The listing builds one solid part. Answer for the finished solid, in the listing's coordinates (mm). A direction names the side the tool comes from. Round coordinates to 2 decimals unless told otherwise and drop trailing zeros. Write each loop counter-clockwise with the first axis right and the second up, starting at its lowest first coordinate (ties: lowest second). Pieces come first, ordered by that corner, then holes. Notation, with made-up numbers: (89.25, 46.25) - (116.25, 46.25) arc R24 cw to (116.25, 74.25) - close; hole circle Ø2 at (68, -16.5). An arc over 180 degrees is marked (long way). Answer as CSV lines item,"result". Start each with the question number.
Item 1: For a pull along Y with two mould halves and no side action, classify faces 1 (the flat face through (-26, 76.809, 1)), 2 (the cylindrical face through (-18.75, 30.73, 4.5)), 3 (the cylindrical face through (-23.75, 24.89, 4.5)) as pulls with the +Y half, pulls with the -Y half, needs draft (parallel to the pull), parting line crosses it, or undercut.
Item 2: Flat-ended cylindrical pins translate along their axes: pin 1 (2 mm diameter, centred on x = -15.5, z = 1, fed in from +Y); pin 2 (4 mm diameter, centred on x = -21.25, y = 26.81, fed in from +Z); pin 3 (4 mm diameter, centred on x = -16, y = 59, fed in from -Z); pin 4 (1.5 mm diameter, centred on x = -14.5, z = 1.5, fed in from +Y). Find the tip coordinate at first contact, or state that the pin passes through.
Item 3: A cutting plane is placed at A-A on y = 60. Determine the outline of the cut face in (x, z), and give its area (3 significant figures).
Item 4: Straight lines are drawn through the part: line 1 along Y through (x, z) = (-21.25, 2.3); line 2 along Y through (x, z) = (-21.25, 4.75); line 3 along Y through (x, z) = (-20, 1.25). For each, find the intervals that lie inside material, in ascending order. Write a range as [from, to].
Item 5: A cutting plane is placed at B-B on x = -14. Determine the outline of the cut face in (y, z).
Item 6: Which of the six approach directions +Z, -Z, +X, -X, +Y, -Y give full straight-line access (tool end or side, diameter ignored) to faces 4 (the cylindrical face through (-21.47, 16.81, 1.48)), 5 (the flat face through (-23, 26, 3))?
```python
from build123d import *

# Parameters (mm, degrees)
BOSS_EXTRUDE1_DEPTH = 3
SKETCH2_R           = 4.65
SKETCH2_R_2         = 3.15
BOSS_EXTRUDE2_DEPTH = 3.044394089
SKETCH3_R           = 1.575
CUT_EXTRUDE1_DEPTH  = 6.044394089
SKETCH4_R           = 1.575
CUT_EXTRUDE2_DEPTH  = 12


with BuildPart() as part:
    # Sketch1 → Boss-Extrude1 (new body)
    with BuildSketch(Plane.XY):
        with BuildLine():
            Line((-31.25, 76.808826039), (-31.25, 26.808826039))
            ThreePointArc((-31.25, 26.808826039), (-21.25, 16.808826039), (-11.25, 26.808826039))
            Line((-11.25, 26.808826039), (-11.25, 66.808826039))
            ThreePointArc((-11.25, 66.808826039), (-14.178932188, 73.879893851), (-21.25, 76.808826039))
            Line((-21.25, 76.808826039), (-31.25, 76.808826039))
        make_face()
    extrude(amount=BOSS_EXTRUDE1_DEPTH)

    # Sketch2 → Boss-Extrude2 (add)
    with BuildSketch(Plane.XY.offset(3)):
        with Locations((-21.25, 26.808826039)):
            Circle(SKETCH2_R)
        with Locations((-21.25, 26.808826039)):
            Circle(SKETCH2_R_2, mode=Mode.SUBTRACT)
    extrude(amount=BOSS_EXTRUDE2_DEPTH)

    # Sketch3 → Cut-Extrude1 (cut)
    with BuildSketch(Plane(origin=(0, 0, 0), x_dir=(-1, 0, 0), z_dir=(0, 0, -1))):
        with Locations((21.25, 26.808826039)):
            Circle(SKETCH3_R)
    extrude(amount=-CUT_EXTRUDE1_DEPTH, mode=Mode.SUBTRACT)

    # Sketch4 → Cut-Extrude2 (cut)
    with BuildSketch(Plane(origin=(0, 0, 0), x_dir=(-1, 0, 0), z_dir=(0, 0, -1))):
        with Locations((21.25, 66.808826039)):
            Circle(SKETCH4_R)
    extrude(amount=-CUT_EXTRUDE2_DEPTH, mode=Mode.SUBTRACT)


solid = part.part
```
Geometry says:
1,face 1,"pulls with the +Y half"
1,face 2,"parting line crosses it"
1,face 3,"undercut"
2,pin 1,"stops at y = 75.61"
2,pin 2,"stops at z = 3"
2,pin 3,"stops at z = 0"
2,pin 4,"stops at y = 74.81"
3,outline,"(-31.25, 0) - (-11.25, 0) - (-11.25, 3) - (-31.25, 3) - close"
3,area,"60.0 mm^2"
4,line 1,"y = [16.81, 25.23], [28.38, 65.23], [68.38, 76.81]"
4,line 2,"y = [22.16, 23.66], [29.96, 31.46]"
4,line 3,"y = [16.89, 25.85], [27.77, 65.85], [67.77, 76.73]"
5,outline,"(19.92, 0) - (73.7, 0) - (73.7, 3) - (19.92, 3) - close"
6,face 4,"+Z, -Z, -Y"
6,face 5,"+Z"
